```python
from build123d import *


with BuildPart() as f5:
    # F4 (on Front) → F5 (revolve)
    with BuildSketch(Plane.XZ):
        with BuildLine():
            Line((0, 16.9418), (0, 0))
            Line((0, 0), (0, -8.4582))
            ThreePointArc((0, -8.4582), (25.4, 16.9418), (0, 42.3418))
            Line((0, 42.3418), (0, 16.9418))
        make_face()
    revolve(axis=Axis((0, 0, 16.9418), (0, 0, -1)))

    # F2 (on Top) → F6 (revolve, intersect)
    with BuildSketch(Plane.XY):
        with BuildLine():
            Line((0, 46.263021417), (0, -12.2905196622))
            ThreePointArc((0, -12.2905196622), (29.2767705396, 16.9862508774), (0, 46.263021417))
        make_face()
    revolve(axis=Axis((0, 16.9862508774, 0), (0, -1, 0)), mode=Mode.INTERSECT)

    # F3 (on Top) → F8 (revolve, intersect)
    with BuildSketch(Plane.XY):
        with BuildLine():
            Line((-39.9929191695, -22.8585096233), (10.7572382071, 6.4421073995))
            ThreePointArc((10.7572382071, 6.4421073995), (-29.2681489926, 17.1668775764), (-39.9929191695, -22.8585096233))
        make_face()
    revolve(axis=Axis((-14.6178404812, -8.2082011119, 0), (-0.8660254038, -0.5, 0)), mode=Mode.INTERSECT)

    # F1 (on Top) → F9 (revolve, intersect)
    with BuildSketch(Plane.XY):
        with BuildLine():
            Line((0, -0.0084829462), (0, 0))
            Line((0, 0), (-10.7133459402, 6.179514724))
            ThreePointArc((-10.7133459402, 6.179514724), (0.0151414181, -33.805722394), (39.9988528315, -23.0715503257))
            Line((39.9988528315, -23.0715503257), (14.6406725481, -8.4448175281))
            Line((14.6406725481, -8.4448175281), (0.0073489014, -0.0042388853))
            Line((0.0073489014, -0.0042388853), (0, -0.0084829462))
        make_face()
    revolve(axis=Axis((14.6427534456, -8.4460178008, 0), (0.8662297429, -0.4996459071, 0)), mode=Mode.INTERSECT)


solid = f5.part
```
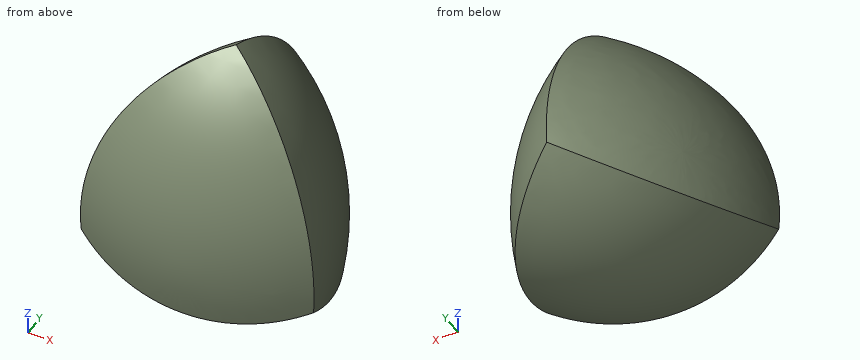
Input: part model. Units: mm. Frame: model coordinates. Coordinates: 2 decimals unless noted, no trailing zeros. Loops run counter-clockwise (first coordinate to the right, second up) from the corner with the lowest first, then second, coordinate; pieces in that order, holes last. Notation, with made-up numbers: (50.25, 2) - (57.25, 2) arc R8 ccw to (57.25, 15) - close; hole circle Ø11 at (42.5, 40.5). An arc over 180 degrees is marked (long way). Answer in a Markdown table with one row per item.
(1) Cut plane B-B on x = 12. Output: boundary loops of the cut face in (y, z).
Model answer:
| item | result |
|---|---|
| outline | (-9.51, -3.32) arc R22.39 ccw to (2.85, -5.26) arc R12.25 ccw to (-6.79, 12.17) arc R26.7 ccw to start |
(2) Material intervals for L1, parallel to X at y = 15.5, z = 2; L2, parallel to X at y = 13, z = -2; L3, parallel to Z at x = -5, y = 8.5, sorted ascending. Write a range as from..to.
Model answer:
| item | result |
|---|---|
| L1 | x = -2.08..2.48 |
| L2 | x = -5.18..5.5 |
| L3 | z = -6.47..13.56 |
(3) Pin query (flat end, axial travel): P1, Ø3, axis at y = -9, z = -2, coming from the +X side; P2, Ø6, axis at y = 8.5, z = 20, coming from the +X side; P3, Ø6, axis at x = 9.5, z = -3, coming from the +Y side. Return the tip coordinate at first contact, or that it passes through.
Model answer:
| item | result |
|---|---|
| P1 | stops at x = 14.68 |
| P2 | stops at x = 3.46 |
| P3 | stops at y = 11.91 |
(4) Cut plane A-A on x = 8. Output: boundary loops of the cut face in (y, z), plus the area to 3 significant figures.
Model answer:
| item | result |
|---|---|
| outline | (-10.8, -4.61) arc R24.11 ccw to (9.7, -5.13) arc R18.63 ccw to (-4.47, 18.25) arc R28.16 ccw to start |
| area | 422 mm² |
